Model file for the job. Use its own axes, mm. Face numbers are marked on the shaded views. A direction names the side the tool comes from. Give positions to 0.01 mm unless a question says otherwise; leave off trailing zeros. Loops run counter-clockwise (first coordinate to the right, second up) from the corner with the lowest first, then second, coordinate; pieces in that order, holes last. Notation, with made-up numbers: M 11.25,-15 L 63.25,-15 A18 ccw 63.25,15 Z; hole C 57,61.5 d9. An arc over 180 degrees is marked long. Answer in a Markdown table with one row per item.
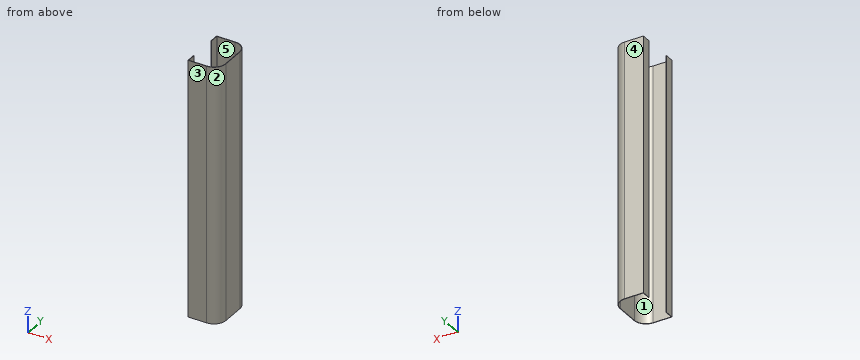
Autodesk Inventor part; units mm, degrees
ref_plane "YZ Plane" through (0, 0, 0) normal (1, 0, 0) x (0, 1, 0)
ref_plane "XZ Plane" through (0, 0, 0) normal (0, 1, 0) x (-1, 0, 0)
ref_plane "XY Plane" through (0, 0, 0) normal (0, 0, 1) x (1, 0, 0)
sketch "Sketch1" plane through (0, 0, 0) normal (0, 0, 1) x (1, 0, 0)
  line L0 (0, 0) -> (19.05, 0) construction
  line L1 (19.05, 0) -> (19.05, 127) construction
  line L2 (19.05, 127) -> (0, 127) construction
  line L3 (0, 127) -> (0, 0) construction
  line L4 (19.05, 127) -> (82.55, 127) construction
  line L5 (82.55, 127) -> (82.55, 0) construction
  line L6 (82.55, 0) -> (19.05, 0) construction
  line L7 (19.05, 0) -> (19.05, 127) construction
  line L8 (0, 127) -> (50.8, 127)
  line L9 (50.8, 127) -> (50.8, 128.27)
  line L10 (50.8, 128.27) -> (0, 128.27)
  line L11 (0, 128.27) -> (0, 127)
  line L12 (0, 0) -> (50.8, 0)
  line L13 (50.8, 0) -> (50.8, -1.27)
  line L14 (50.8, -1.27) -> (0, -1.27)
  line L15 (0, -1.27) -> (0, 0)
  arc A0 (50.8, 0) -> (82.55, 31.75) centre (50.8, 31.75) ccw
  line L16 (50.8, 0) -> (82.55, 31.75) construction
  line L17 (50.8, 0) -> (95.7013, 0) construction
  arc A1 (82.55, 95.25) -> (50.8, 127) centre (50.8, 95.25) ccw
  line L18 (50.8, 127) -> (82.55, 95.25) construction
  line L19 (50.8, 127) -> (95.7013, 127) construction
  line L20 (82.55, 95.25) -> (83.82, 95.25)
  line L21 (83.82, 95.25) -> (83.82, 31.75)
  line L22 (83.82, 31.75) -> (82.55, 31.75)
  line L23 (82.55, 31.75) -> (82.55, 95.25)
  arc A2 (83.82, 95.25) -> (50.8, 128.27) centre (50.8, 95.25) ccw
  arc A3 (50.8, -1.27) -> (83.82, 31.75) centre (50.8, 31.75) ccw
  line L24 (82.55, 31.75) -> (83.82, 31.75)
  dimension "d0" = 19.05
  dimension "d1" = 127
  dimension "d2" = 63.5
  dimension "d3" = 127
  dimension "d4" = 50.8
  dimension "d5" = 1.27
  dimension "d6" = 50.8
  dimension "d7" = 1.27
  dimension "d8" = 45
  dimension "d9" = 31.75
  dimension "d10" = 45
  dimension "d11" = 31.75
  dimension "d12" = 1.27
  dimension "d13" = 63.5
  dimension "d14" = 33.02
  dimension "d15" = 33.02
extrude "Extrusion1" add sketch "Sketch1" along normal blind 711.2
sketch "Sketch2" plane through (0, 0, 711.2) normal (0, 0, 1) x (1, 0, 0)
  line L0 (50.8, 128.27) -> (0, 128.27)
  line L1 (0, 128.27) -> (0, 127)
  line L2 (0, 127) -> (50.8, 127)
  arc A0 (82.55, 95.25) -> (50.8, 127) centre (50.8, 95.25) ccw
  line L3 (82.55, 95.25) -> (82.55, 31.75)
  arc A1 (50.8, 0) -> (82.55, 31.75) centre (50.8, 31.75) ccw
  line L4 (50.8, 0) -> (0, 0)
  line L5 (0, 0) -> (0, -1.27)
  line L6 (0, -1.27) -> (50.8, -1.27)
  arc A2 (50.8, -1.27) -> (83.82, 31.75) centre (50.8, 31.75) ccw
  line L7 (83.82, 31.75) -> (83.82, 95.25)
  arc A3 (83.82, 95.25) -> (50.8, 128.27) centre (50.8, 95.25) ccw
  line L8 (0, 128.27) -> (-1.27, 128.27)
  line L9 (-1.27, 128.27) -> (-1.27, 102.87)
  line L10 (-1.27, 102.87) -> (0, 102.87)
  line L11 (0, 102.87) -> (0, 128.27)
  line L12 (0, -1.27) -> (-1.27, -1.27)
  line L13 (-1.27, -1.27) -> (-1.27, 24.13)
  line L14 (-1.27, 24.13) -> (0, 24.13)
  line L15 (0, 24.13) -> (0, -1.27)
  dimension "d18" = 1.27
  dimension "d19" = 25.4
  dimension "d20" = 1.27
  dimension "d21" = 25.4
extrude "Extrusion2" add sketch "Sketch2" against normal blind 711.2 contours L1 L11 L10 L9 L8 | L12 L13 L14 L15 L5
properties part number "bumper_cloth"
(1) Saw through at A-A, the plane x = 8. Give the cut face in (y, z).
Established:
| item | result |
|---|---|
| outline | M -1.27,0 L 0,0 L 0,711.2 L -1.27,711.2 Z; M 127,0 L 128.27,0 L 128.27,711.2 L 127,711.2 Z |
(2) Saw through at B-B, the plane y = 8.5. Give the cut face in (x, z).
Established:
| item | result |
|---|---|
| outline | M -1.27,0 L 0,0 L 0,711.2 L -1.27,711.2 Z; M 72.42,0 L 74.25,0 L 74.25,711.2 L 72.42,711.2 Z |
(3) Saw through at D-D, the plane y = 40. Give the cut face in (x, z), and give its area (3 significant figures).
Established:
| item | result |
|---|---|
| outline | M 82.55,0 L 83.82,0 L 83.82,711.2 L 82.55,711.2 Z |
| area | 903 mm2 |
(4) Saw through at C-C, the plane z = 121.5. Give the cut face in (x, y).
Established:
| item | result |
|---|---|
| outline | M -1.27,-1.27 L 50.8,-1.27 A33.02 ccw 83.82,31.75 L 83.82,95.25 A33.02 ccw 50.8,128.27 L -1.27,128.27 L -1.27,102.87 L 0,102.87 L 0,127 L 50.8,127 A31.75 cw 82.55,95.25 L 82.55,31.75 A31.75 cw 50.8,0 L 0,0 L 0,24.13 L -1.27,24.13 Z |
(5) Which spindle directions (+Z, -Z, +X, -X, +Y, -Y) get a long thin tool onto all of the face, cutting with end or side? Do the marked faces 4 and 5. Say none if no direction does.
Established:
| item | result |
|---|---|
| face 4 | +Z, -Z, +X, -X, +Y |
| face 5 | +Z, -Z |
(6) Mould opens along X. For the marked faces 1, 2 and 3 say: pulls with the +X half, pulls with the -X half, needs draft (parallel to the pull), parting line crosses it, or undercut.
Established:
| item | result |
|---|---|
| face 1 | undercut |
| face 2 | pulls with the +X half |
| face 3 | needs draft |
(7) Flat gauge pins, fed straight in: P1, Ø12, axis at y = 116.5, z = 510.5, coming from the +X side; P2, Ø7, axis at y = 9.5, z = 493, coming from the +X side; P3, Ø1.5, axis at x = 70.5, z = 566.5, coming from the -Y side. Where does each tip first touch, or does it go through?
Established:
| item | result |
|---|---|
| P1 | stops at x = 80.09 |
| P2 | stops at x = 77.98 |
| P3 | stops at y = 4.71 |
(8) Wall check: L1, parallel to Y at x = 21.5, z = 669; L2, parallel to Y at x = 52, z = 558; L3, parallel to X at y = 66, z = 325. Give the ranges that are in metal, low to high.
Established:
| item | result |
|---|---|
| L1 | y = -1.27 to 0, 127 to 128.27 |
| L2 | y = -1.25 to 0.02, 126.98 to 128.25 |
| L3 | x = 82.55 to 83.82 |
